from build123d import *

# Parameters (mm, degrees)
SKETCH1_R               = 1.5
SKETCH1_R_2             = 11.5
BOSS_EXTRUDE1_DEPTH     = 5
BOSS_EXTRUDE2_DEPTH     = 54
CUT_EXTRUDE1_DEPTH      = 64.518855468
CUT_EXTRUDE1_DEPTH_BACK = 64.518855468
FILLET1_R               = 10
BOSS_EXTRUDE3_DEPTH     = 51
CHAMFER2_SIZE           = 1
BOSS_EXTRUDE4_DEPTH     = 54
CHAMFER3_SIZE           = 1
CHAMFER4_SIZE           = 1
CHAMFER5_SIZE           = 1
SKETCH11_R              = 4
CUT_EXTRUDE2_DEPTH      = 3
SKETCH12_R              = 2
CUT_EXTRUDE3_DEPTH      = 73.557649493
CHAMFER6_SIZE           = 1


with BuildPart() as part:
    # Sketch1 → Boss-Extrude1 (new body)
    with BuildSketch(Plane(origin=(0, 0, 0), x_dir=(1, 0, 0), z_dir=(0, 1, 0))):
        Polygon((-21.15, 17.15), (-17.15, 21.15), (17.15, 21.15), (21.15, 17.15), (21.15, -17.15), (17.15, -21.15), (-17.15, -21.15), (-21.15, -17.15), align=None)
        with Locations(Location((-15.5, 15.5, 0), (0, 0, 270))):
            Circle(SKETCH1_R, mode=Mode.SUBTRACT)
        with Locations(Location((15.5, 15.5, 0), (0, 0, 270))):
            Circle(SKETCH1_R, mode=Mode.SUBTRACT)
        with Locations(Location((15.5, -15.5, 0), (0, 0, 270))):
            Circle(SKETCH1_R, mode=Mode.SUBTRACT)
        with Locations(Location((-15.5, -15.5, 0), (0, 0, 270))):
            Circle(SKETCH1_R, mode=Mode.SUBTRACT)
        with Locations(Location((0, 0, 0), (0, 0, 270))):
            Circle(SKETCH1_R_2, mode=Mode.SUBTRACT)
    extrude(amount=BOSS_EXTRUDE1_DEPTH)

    # Sketch5 → Boss-Extrude2 (add)
    with BuildSketch(Plane(origin=(0, 0, 0), x_dir=(1, 0, 0), z_dir=(0, 1, 0))):
        Polygon((-23.65, 14.65), (-23.65, -18.185533906), (-18.185533906, -23.65), (18.185533906, -23.65), (23.65, -18.185533906), (23.65, 14.65), (21.15, 17.15), (21.15, -17.15), (17.15, -21.15), (-17.15, -21.15), (-21.15, -17.15), (-21.15, 17.15), align=None)
    extrude(amount=BOSS_EXTRUDE2_DEPTH)

    # Sketch6 → Cut-Extrude1 (cut, two sides: drawn at the far end of the back side and taken through both)
    with BuildSketch(Plane(origin=(0, 0, 0), x_dir=(0, 0, -1), z_dir=(1, 0, 0)).offset(-CUT_EXTRUDE1_DEPTH_BACK)):
        Polygon((17.15, 5), (-18.15, 40.3), (-18.15, 54), (17.15, 54), align=None)
    extrude(amount=CUT_EXTRUDE1_DEPTH + CUT_EXTRUDE1_DEPTH_BACK, mode=Mode.SUBTRACT)

    # Fillet1
    fillet1_edges = [part.edges().sort_by_distance(p)[0] for p in [
        (-21.9, 40.3, 18.15),
        (21.9, 40.3, 18.15),
    ]]
    fillet(fillet1_edges, radius=FILLET1_R)

    # Sketch9 → Boss-Extrude3 (add)
    with BuildSketch(Plane(origin=(0, 0, 0), x_dir=(1, 0, 0), z_dir=(0, 1, 0))):
        Polygon((-18.185533906, -23.65), (-21, -28.524798271), (21, -28.524798271), (18.185533906, -23.65), align=None)
    extrude(amount=BOSS_EXTRUDE3_DEPTH)

    # Chamfer2
    chamfer2_edges = [part.edges().sort_by_distance(p)[0] for p in [
        (0, 0, -11.5),
    ]]
    chamfer(chamfer2_edges, length=CHAMFER2_SIZE)

    # Sketch10 → Boss-Extrude4 (add)
    with BuildSketch(Plane(origin=(0, 54, 0), x_dir=(1, 0, 0), z_dir=(0, 1, 0))):
        Polygon((-23.65, -18.15), (-20.15, -18.15), (-17.15, -21.15), (17.15, -21.15), (20.15, -18.15), (23.65, -18.15), (23.65, -28.524798271), (-23.65, -28.524798271), align=None)
    extrude(amount=-BOSS_EXTRUDE4_DEPTH)

    # Chamfer3
    chamfer3_edges = [part.edges().sort_by_distance(p)[0] for p in [
        (-23.65, 0, 6.937399136),
        (23.65, 0, 6.937399136),
        (-20.4, 0, -17.9),
        (0, 0, -21.15),
        (20.4, 0, -17.9),
    ]]
    chamfer(chamfer3_edges, length=CHAMFER3_SIZE)

    # Chamfer4
    chamfer4_edges = [part.edges().sort_by_distance(p)[0] for p in [
        (-23.65, 22.435533906, 0.285533906),
        (23.65, 22.435533906, 0.285533906),
        (-23.65, 40.6153013, 17.388795325),
        (23.65, 40.6153013, 17.388795325),
        (-23.65, 49.221067812, 18.15),
        (23.65, 49.221067812, 18.15),
    ]]
    chamfer(chamfer4_edges, length=CHAMFER4_SIZE)

    # Chamfer5
    chamfer5_edges = [part.edges().sort_by_distance(p)[0] for p in [
        (-23.65, 54, 23.837399136),
        (-21.4, 54, 18.15),
        (23.15, 54, 18.65),
        (-23.15, 54, 18.65),
        (23.65, 54, 23.837399136),
        (0, 54, 21.15),
        (-18.65, 54, 19.65),
        (18.65, 54, 19.65),
        (21.4, 54, 18.15),
    ]]
    chamfer(chamfer5_edges, length=CHAMFER5_SIZE)

    # Sketch11 → Cut-Extrude2 (cut)
    with BuildSketch(Plane(origin=(0, 0, 21.15), x_dir=(-1, 0, 0), z_dir=(0, 0, -1))):
        with Locations((-10, 42)):
            Circle(SKETCH11_R)
        with Locations((10, 42)):
            Circle(SKETCH11_R)
        with Locations((-10, 12)):
            Circle(SKETCH11_R)
        with Locations((10, 12)):
            Circle(SKETCH11_R)
    extrude(amount=-CUT_EXTRUDE2_DEPTH, mode=Mode.SUBTRACT)

    # Sketch12 → Cut-Extrude3 (cut, through all)
    with BuildSketch(Plane(origin=(0, 0, 21.15), x_dir=(-1, 0, 0), z_dir=(0, 0, -1))):
        with Locations((-10, 42)):
            Circle(SKETCH12_R)
        with Locations((10, 42)):
            Circle(SKETCH12_R)
        with Locations((-10, 12)):
            Circle(SKETCH12_R)
        with Locations((10, 12)):
            Circle(SKETCH12_R)
    extrude(amount=-CUT_EXTRUDE3_DEPTH, mode=Mode.SUBTRACT)

    # Chamfer6
    chamfer6_edges = [part.edges().sort_by_distance(p)[0] for p in [
        (-6, 42, 21.15),
        (14, 12, 21.15),
        (-6, 12, 21.15),
        (14, 42, 21.15),
    ]]
    chamfer(chamfer6_edges, length=CHAMFER6_SIZE)


solid = part.part
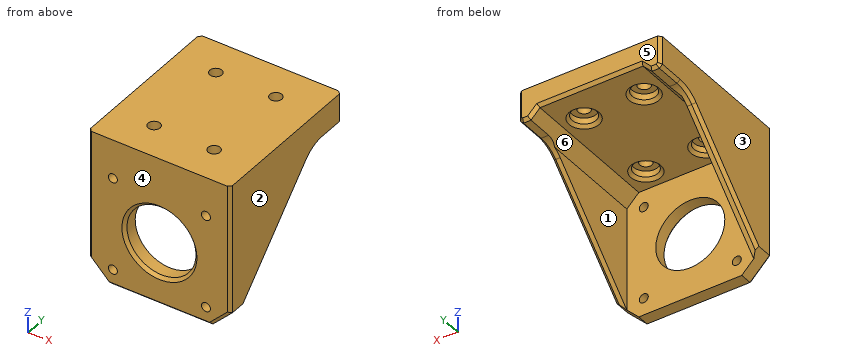
Input: part model. Units: mm. Frame: model coordinates. Face numbers are marked on the shaded views. A direction names the side the tool comes from. Round coordinates to 2 decimals unless told otherwise and drop trailing zeros. Loops run counter-clockwise (first coordinate to the right, second up) from the corner with the lowest first, then second, coordinate; pieces in that order, holes last. Notation, with made-up numbers: (58.5, 50.25) -> (103.5, 50.25) arc R22 ccw to (103.5, 76.25) -> close; hole circle Ø5 at (43, 60.5). An arc over 180 degrees is marked (long way). Answer as a JSON object with one key per item and string values. Group by question number.
1) Reachability of the marked faces 5 and 6 from +Z, -Z, +X, -X, +Y, -Y: full face, straight path, thin tool, end or side. Return the list, or none.
2) Section query B-B on z = 0. Output: boundary loops of the cut face in (x, y), plus the area to 3 significant figures.
3) Section query C-C on y = 26. Output: boundary loops of the cut face in (x, z).
4) Draft query along X for the marked faces 1, 2, 3 and 4. Return one class per face: +X half, -X half, draft (parallel to the pull), parting line (faces both ways), or undercut.
5) Section query A-A on y = 12. State how many separate pieces and enclosed holes the cut face has, plus the area to 3 significant figures.
6) Pin query (flat end, axial travel): pin 1 (4 mm diameter, centred on x = 9.5, y = 42.5, fed in from -Z); pin 2 (3 mm diameter, centred on x = 21.5, y = 48, fed in from -Z); pin 3 (2 mm diameter, centred on x = -21.5, y = 48.5, fed in from -Z); pin 4 (2.5 mm diameter, centred on x = 15.5, z = -15.5, fed in from +Y). Return the tip coordinate at first contact, or that it passes through.
7) Ray query, L1, parallel to Y at x = -10, z = 22.65; L2, parallel to Y at x = 10, z = 25.85; L3, parallel to Z at x = -4, y = 14.5. Return the intervals inside material, ascending.
Reply:
{
 "1": {"face 5": "+Z, -Z, +X, -X, +Y", "face 6": "-Z, +Y"},
 "2": {"outline": "(-23.65, 1) -> (-22.65, 0) -> (-12.5, 0) -> (-11.5, 1) -> (-11.5, 5) -> (-21.15, 5) -> (-21.15, 22.15) -> (-22.65, 22.15) -> (-23.65, 20.74) -> close; (11.5, 1) -> (12.5, 0) -> (22.65, 0) -> (23.65, 1) -> (23.65, 20.74) -> (22.65, 22.15) -> (21.15, 22.15) -> (21.15, 5) -> (11.5, 5) -> close", "area": "204 mm2"},
 "3": {"outline": "(-23.65, 5.26) -> (-22.65, 3.85) -> (-21.15, 3.85) -> (-21.15, 17.15) -> (-17.15, 21.15) -> (17.15, 21.15) -> (21.15, 17.15) -> (21.15, 3.85) -> (22.65, 3.85) -> (23.65, 5.26) -> (23.65, 28.52) -> (-23.65, 28.52) -> close"},
 "4": {"face 1": "undercut", "face 2": "+X half", "face 3": "-X half", "face 4": "draft"},
 "5": {"separate pieces": "3", "enclosed holes": "0", "area": "435 mm2"},
 "6": {"pin 1": "stops at z = 24.15", "pin 2": "stops at z = 18.15", "pin 3": "stops at z = 18.15", "pin 4": "passes through"},
 "7": {"L1": "y = 0 to 8, 16 to 38, 46 to 54", "L2": "y = 0 to 10, 14 to 40, 44 to 54", "L3": "z = 21.15 to 28.52"}
}
